Check sheet for the modelled part. Datum: model origin and axes. Units: mm. Coordinates: 2 decimals unless noted, no trailing zeros. Loops run counter-clockwise (first coordinate to the right, second up) from the corner with the lowest first, then second, coordinate; pieces in that order, holes last. Notation, with made-up numbers: M -11.5,-7.5 L 27.5,-7.5 A15 cw 27.5,8.5 Z; hole C -36,83 d8. An arc over 180 degrees is marked long. Use CSV: the item, a comma, the result in double quotes. Start each with the question number.
(1) Section check A-A on z = 22.75. Record the cut outline in (x, y).
(2) Scan lines: line 1 (X direction, y = -5.5, z = 5); line 2 (Y direction, x = -81.5, z = 4.75); line 3 (Y direction, x = -68, z = 4.25). Record each from-to range of solid material in increasing order.
(3) Draft check along Z on faces 1 (the cylindrical face through (38.581, -10.397, 23.872)), 2 (the cylindrical face through (-27.03, 33.58, 1.53)), 3 (the cylindrical face through (38.5, 33.58, 12.81)). Enter one of: pulls with the +Z half, pulls with the -Z half, needs draft (parallel to the pull), parting line crosses it, or undercut.
(4) Go/stop test with a flat-tipped pin: pin 1 Ø2 at (y, z) = (4, 3) entering from -X. Record where the tip stops, or that it passes through.
from build123d import *

# Parameters (mm, degrees)
F1_DEPTH = 25.4
F2_R     = 5.08


with BuildPart() as f1:
    # F0 (on Top) → F1 (new body)
    with BuildSketch(Plane.XY):
        with BuildLine():
            Line((40.0298386812, 35.026114434), (-92.3765525222, 35.026114434))
            Line((-92.3765525222, 35.026114434), (-92.3765525222, 0))
            Line((-92.3765525222, 0), (-54.1899020415, 0))
            ThreePointArc((-54.1899020415, 0), (-29.6374764293, 14.3361382619), (-5.0850508172, 0))
            Line((-5.0850508172, 0), (40.0298386812, 0))
            Line((40.0298386812, 0), (40.0298386812, 35.026114434))
        make_face()
        with BuildLine():
            Line((-54.1899020415, 0), (-92.3765525222, 0))
            Line((-92.3765525222, 0), (-92.3765525222, -30.0223715603))
            Line((-92.3765525222, -30.0223715603), (-52.7348229784, -30.0223715603))
            ThreePointArc((-52.7348229784, -30.0223715603), (-57.7970377768, -15.2212722889), (-54.1899020415, 0))
        make_face()
        with BuildLine():
            Line((40.0298386812, -30.0223715603), (40.0298386812, 0))
            Line((40.0298386812, 0), (-5.0850508172, 0))
            ThreePointArc((-5.0850508172, 0), (-2.3700906657, -6.6931514243), (-1.4448610633, -13.8564771041))
            ThreePointArc((-1.4448610633, -13.8564771041), (-2.7488341392, -22.3314093736), (-6.5401298802, -30.0223715603))
            Line((-6.5401298802, -30.0223715603), (40.0298386812, -30.0223715603))
        make_face()
        with BuildLine():
            Line((-52.7348229784, -30.0223715603), (-92.3765525222, -30.0223715603))
            Line((-92.3765525222, -30.0223715603), (-92.3765525222, -56.965533644))
            Line((-92.3765525222, -56.965533644), (40.0298386812, -56.965533644))
            Line((40.0298386812, -56.965533644), (40.0298386812, -30.0223715603))
            Line((40.0298386812, -30.0223715603), (-6.5401298802, -30.0223715603))
            ThreePointArc((-6.5401298802, -30.0223715603), (-29.6374764293, -42.0490924702), (-52.7348229784, -30.0223715603))
        make_face()
        with BuildLine():
            ThreePointArc((-5.0850508172, 0), (-29.6374764293, 14.3361382619), (-54.1899020415, 0))
            Line((-54.1899020415, 0), (-26.1733569205, 0))
            Line((-26.1733569205, 0), (-5.0850508172, 0))
        make_face()
        with BuildLine():
            Line((-26.1733569205, 0), (-54.1899020415, 0))
            ThreePointArc((-54.1899020415, 0), (-57.7970377768, -15.2212722889), (-52.7348229784, -30.0223715603))
            Line((-52.7348229784, -30.0223715603), (-6.5401298802, -30.0223715603))
            ThreePointArc((-6.5401298802, -30.0223715603), (-2.7488341392, -22.3314093736), (-1.4448610633, -13.8564771041))
            ThreePointArc((-1.4448610633, -13.8564771041), (-2.3700906657, -6.6931514243), (-5.0850508172, 0))
            Line((-5.0850508172, 0), (-26.1733569205, 0))
        make_face()
        with BuildLine():
            Line((-6.5401298802, -30.0223715603), (-52.7348229784, -30.0223715603))
            ThreePointArc((-52.7348229784, -30.0223715603), (-29.6374764293, -42.0490924702), (-6.5401298802, -30.0223715603))
        make_face()
    extrude(amount=F1_DEPTH)

    # F2
    f2_edges = [f1.edges().sort_by_distance(p)[0] for p in [
        (40.029839, -56.965534, 12.7),
        (40.029839, 35.026114, 12.7),
        (40.029839, -10.96971, 0),
        (40.029839, -10.96971, 25.4),
        (-92.376553, -56.965534, 12.7),
        (-26.173357, -56.965534, 0),
        (-26.173357, -56.965534, 25.4),
        (-92.376553, 35.026114, 12.7),
        (-26.173357, 35.026114, 0),
        (-26.173357, 35.026114, 25.4),
        (-92.376553, -10.96971, 0),
        (-92.376553, -10.96971, 25.4),
    ]]
    fillet(f2_edges, radius=F2_R)


solid = f1.part
Outcome:
1,outline,"M -91.76,-51.89 A4.46 ccw -87.3,-56.35 L 34.95,-56.35 A4.46 ccw 39.41,-51.89 L 39.41,29.95 A4.46 ccw 34.95,34.41 L -87.3,34.41 A4.46 ccw -91.76,29.95 Z"
2,line 1,"x = -92.38 to 40.03"
2,line 2,"y = -56.95 to 35.02"
2,line 3,"y = -56.9 to 34.96"
3,face 1,"pulls with the +Z half"
3,face 2,"pulls with the -Z half"
3,face 3,"needs draft"
4,pin 1,"stops at x = -92.26"
